Autodesk Inventor part; units mm, degrees
ref_plane "Work Plane1" through (-8.7167, 0, 0) normal (0, 0, -1) x (1, 0, 0)
ref_plane "YZ Plane" through (0, 0, 0) normal (1, 0, 0) x (0, 1, 0)
ref_plane "XZ Plane" through (0, 0, 0) normal (0, 1, 0) x (-1, 0, 0)
sketch "Schizzo1" plane through (0, 0, 0) normal (1, 0, 0) x (0, 1, 0)
  line L0 (2.0207, -3.5) -> (-2.0207, -3.5)
  line L1 (-2.0207, -3.5) -> (-4.0415, 0)
  line L2 (-4.0415, 0) -> (-2.0207, 3.5)
  line L3 (-2.0207, 3.5) -> (2.0207, 3.5)
  line L4 (2.0207, 3.5) -> (4.0415, 0)
  line L5 (4.0415, 0) -> (2.0207, -3.5)
  point P0 (0, 0)
  point P1 (0, 0)
  dimension "d0" = 8.0829
extrude "Corpo" add sketch "Schizzo1" along normal blind 2.2
sketch "Schizzo2" plane through (2.2, 0, 0) normal (1, 0, 0) x (0, 0, -1)
  point P0 (0, 0)
hole "Filettatura" at (2.2, 0, 0) direction (-1, 0, 0) diameter 3.242 end through all
chamfer "Smusso2" distance 0.3789 angle 30 1 edges at (2.2, 0, 1.621) measured on face at (2.2, -2.4654, 1.4736)
chamfer "Smusso1" distance 0.3789 angle 30 1 edges at (0, 0, 1.621) measured on face at (0, -2.4654, 1.4736)
ref_plane "Work Plane1" through (-8.7167, 0, 0) normal (0, 0, -1) x (1, 0, 0)
equation "\"d0\" = 1.1547 * SW"
equation "\"d1\" = KOH"
equation "\"d12\" = -0.5 * GD1 + 0.5 * NND"
equation "\"d19\" = -0.5 * GD1 + 0.5 * NND"
equation "\"d10\" = -0.5 * GD1 + 0.5 * NND"
equation "\"d18\" = -0.5 * GD1 + 0.5 * NND"
equation "\"NND\" = 4"
equation "\"KOH\" = 2.2"
equation "\"SW\" = 7"
equation "\"GUL\" = 0.541266 * PTC"
equation "\"THREADDIA\" = 4"
equation "\"TOA\" = 30deg"
equation "\"PTC\" = 0.7"
equation "\"E0\" = 1.155 * SW"
equation "\"GAL\" = 0.541266 * PTC"
properties part number "AS 1474 - M4" material "Acciaio, Dolce"
The listing builds one solid part. Answer for the finished solid, in the listing's coordinates (mm). Coordinates: 2 decimals unless noted, no trailing zeros. Loops run counter-clockwise (first coordinate to the right, second up) from the corner with the lowest first, then second, coordinate; pieces in that order, holes last. Notation, with made-up numbers: (25.5, -29.5) -> (35.5, -29.5) arc R22 cw to (35.5, 2.5) -> close; hole circle Ø7 at (24.25, -17). An arc over 180 degrees is marked (long way). Write item = value, one per line. Start each with the question number.
1) A cutting plane is placed at A-A (y = 0). Give the vertices of the cut face in (x, z).
2) A cutting plane is placed at C-C (z = 3.25). Give the vertices of the cut face in (x, y), then the cut area to 3 significant figures.
3) Given pin 1 Ø1.5 at (y, z) = (0, 1) entering from -X, flat-ended and moving along its own axis, determine where the tip first touches the part or whether it passes through.
4) A cutting plane is placed at D-D (y = 3.25). Give the vertices of the cut face in (x, z), then the cut area to 3 significant figures.
5) A cutting plane is placed at B-B (x = 0.6). Give the vertices of the cut face in (y, z), then the cut area to 3 significant figures.
6) Straight lines are drawn through the part: line 1 (Z direction, x = 1.6, y = 0); line 2 (Y direction, x = 0.3, z = 1.25); line 3 (Y direction, x = 1.95, z = -0.25). For each, find the intervals that lie inside material, in ascending order. Write a range as from..to.
7) The mould has two halves that part along Y. Classify faces 1 (the face through (1.1, -3, -1.8)), 2 (the face through (0, 2, 2)), 3 (the face through (1.088, 1.438, -0.748)): released by +Y, released by -Y, zero draft, split by the parting line, or undercut.
Responses:
q1.outline = (0, -3.5) -> (2.2, -3.5) -> (2.2, -2) -> (1.98, -1.62) -> (0.22, -1.62) -> (0, -2) -> close; (0, 2) -> (0.22, 1.62) -> (1.98, 1.62) -> (2.2, 2) -> (2.2, 3.5) -> (0, 3.5) -> close
q2.outline = (0, -2.17) -> (2.2, -2.17) -> (2.2, 2.17) -> (0, 2.17) -> close
q2.area = 9.53 mm²
q3.pin_1 = 0.14
q4.outline = (0, -1.37) -> (2.2, -1.37) -> (2.2, 1.37) -> (0, 1.37) -> close
q4.area = 6.03 mm²
q5.outline = (-4.04, 0) -> (-2.02, -3.5) -> (2.02, -3.5) -> (4.04, 0) -> (2.02, 3.5) -> (-2.02, 3.5) -> close; hole circle Ø3.24 at (0, 0)
q5.area = 34.2 mm²
q6.line_1 = -3.5..-1.62, 1.62..3.5
q6.line_2 = -3.32..-1.03, 1.03..3.32
q6.line_3 = -3.9..-1.6, 1.6..3.9
q7.face_1 = released by -Y
q7.face_2 = zero draft
q7.face_3 = undercut
